The model under review builds one solid part; all positions refer to its coordinate system, in mm. Face numbers are marked on the shaded views. A direction names the side the tool comes from. Coordinates: 2 decimals unless noted, no trailing zeros. Order: outer loops, then holes, each group sorted by start corner. A loop starts at its lowest first (then second) coordinate and runs counter-clockwise, first axis right, second up. Notation, with made-up numbers: M -40,52.5 L -17,52.5 A27 cw -17,69.5 Z; hole C -33.75,39 d5. An arc over 180 degrees is marked long. Answer in a Markdown table with one row per item.
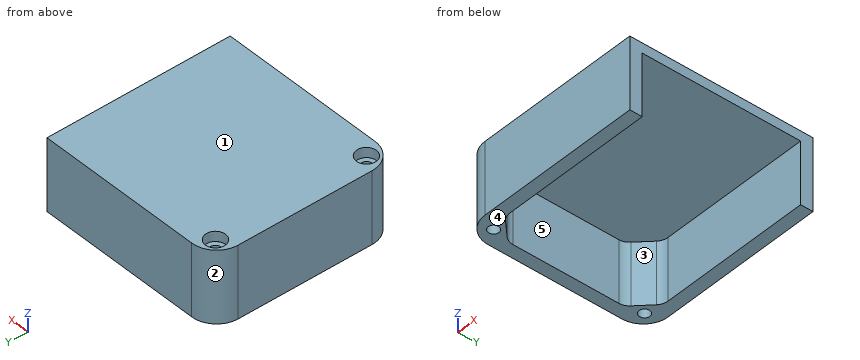
from build123d import *

# Parameters (mm, degrees)
EXTRUDE_THIN1_DEPTH            = 25
BOSS_EXTRUDE1_DEPTH            = 25
SKETCH3_W                      = 76.727105056
SKETCH3_H                      = 73.797041503
BOSS_EXTRUDE2_DEPTH            = 4
FILLET1_R                      = 10
FILLET2_R                      = 5
CBORE_FOR_M4_SHCS1_D           = 4.3
CBORE_FOR_M4_SHCS1_CBORE_D     = 8
CBORE_FOR_M4_SHCS1_CBORE_DEPTH = 4


with BuildPart() as part:
    # Sketch1 → Extrude-Thin1 (new body)
    with BuildSketch(Plane.XY):
        Polygon((-5.007497798, -29.94725217), (-76.734602854, -29.94725217), (-76.734602854, 33.849789333), (-5.007497798, 33.849789333), (-5.007497798, 38.849789333), (-81.734602854, 38.849789333), (-81.734602854, -34.94725217), (-5.007497798, -34.94725217), align=None)
    extrude(amount=EXTRUDE_THIN1_DEPTH)

    # Sketch2 → Boss-Extrude1 (add)
    with BuildSketch(Plane.XY):
        Polygon((-68.24932148, 33.849789333), (-76.734602854, 25.364507959), (-76.734602854, 33.849789333), align=None)
        Polygon((-76.734602854, -29.94725217), (-68.24932148, -29.94725217), (-76.734602854, -21.461970795), align=None)
    extrude(amount=BOSS_EXTRUDE1_DEPTH)

    # Sketch3 → Boss-Extrude2 (add)
    with BuildSketch(Plane.XY.offset(25)):
        with Locations((-43.371050326, 1.951268582)):
            Rectangle(SKETCH3_W, SKETCH3_H)
    extrude(amount=BOSS_EXTRUDE2_DEPTH)

    # Fillet1
    fillet1_edges = [part.edges().sort_by_distance(p)[0] for p in [
        (-81.734602854, -34.94725217, 14.5),
        (-81.734602854, 38.849789333, 14.5),
    ]]
    fillet(fillet1_edges, radius=FILLET1_R)

    # Fillet2
    fillet2_edges = [part.edges().sort_by_distance(p)[0] for p in [
        (-68.24932148, -29.94725217, 12.5),
        (-76.734602854, -21.461970795, 12.5),
        (-68.24932148, 33.849789333, 12.5),
        (-76.734602854, 25.364507959, 12.5),
    ]]
    fillet(fillet2_edges, radius=FILLET2_R)

    # CBORE for M4 SHCS1 (through all)
    with Locations(Plane(origin=(-75.234602854, 32.349789333, 29), x_dir=(1, 0, 0), z_dir=(0, 0, 1))):
        with Locations((0, 0), (0, -60.797041503)):
            CounterBoreHole(CBORE_FOR_M4_SHCS1_D / 2, CBORE_FOR_M4_SHCS1_CBORE_D / 2, CBORE_FOR_M4_SHCS1_CBORE_DEPTH)


solid = part.part
(1) Take a section at A-A (x = -29.5). Write out the cut boundary in (y, z).
Report:
| item | result |
|---|---|
| outline | M -34.95,0 L -29.95,0 L -29.95,25 L 33.85,25 L 33.85,0 L 38.85,0 L 38.85,29 L -34.95,29 Z |
(2) Insertion check: P1, Ø7.5, axis at y = 6.5, z = 18, coming from the +X side; P2, Ø2.5, axis at x = -75.23, y = -28.45, coming from the -Z side; P3, Ø7, axis at x = -75.23, y = -28.45, coming from the +Z side. Each pin has a flat end and moves straight along its axis. Give the tip position at first contact, or say it passes through.
Report:
| item | result |
|---|---|
| P1 | x = -76.73 |
| P2 | through |
| P3 | z = 25 |
(3) Machinability: for the marked faces 4 and 5, which of the approach directions +Z, -Z, +X, -X, +Y, -Y give a long, thin tool a straight path to every point of the face, cutting with its end or side? Answer none if there is none.
Report:
| item | result |
|---|---|
| face 4 | -Z, +X, -X, +Y, -Y |
| face 5 | -Z, +X |
(4) To check wall thickness, follow line 1 (Y direction, x = -14, z = 12); line 2 (Y direction, x = -73.5, z = 16.25); line 3 (Y direction, x = -75, z = 14.5). State the ranges of each line that lie inside material, in increasing order. Write a range as [from, to].
Report:
| item | result |
|---|---|
| line 1 | [-34.95, -29.95], [33.85, 38.85] |
| line 2 | [-34.79, -29.72], [-27.18, -24.7], [28.6, 31.08], [33.62, 38.69] |
| line 3 | [-34.4, -30.58], [-26.31, -23.2], [27.1, 30.21], [34.49, 38.3] |
(5) Take a section at B-B (z = 3.5). Write out the cut boundary in (x, y), then the cut area to 3 significant figures.
Report:
| item | result |
|---|---|
| outline | M -81.73,-24.95 A10 ccw -71.73,-34.95 L -5.01,-34.95 L -5.01,-29.95 L -66.18,-29.95 A5 cw -69.71,-28.48 L -75.27,-22.93 A5 cw -76.73,-19.39 L -76.73,23.29 A5 cw -75.27,26.83 L -69.71,32.39 A5 cw -66.18,33.85 L -5.01,33.85 L -5.01,38.85 L -71.73,38.85 A10 ccw -81.73,28.85 Z; hole C -75.23,-28.45 d4.3; hole C -75.23,32.35 d4.3 |
| area | 1,090 mm^2 |
(6) Take a section at C-C (y = -4). Write out the cut boundary in (x, z), then the cut area to 3 significant figures.
Report:
| item | result |
|---|---|
| outline | M -81.73,0 L -76.73,0 L -76.73,25 L -5.01,25 L -5.01,29 L -81.73,29 Z |
| area | 432 mm^2 |
(7) The part is to be moulded in two halves that separate along Y. For the marked faces 1, 2 and 3, say which applies: +Y half, -Y half, draft (parallel to the pull), parting line (faces both ways), or undercut.
Report:
| item | result |
|---|---|
| face 1 | draft |
| face 2 | +Y half |
| face 3 | undercut |
